```python
from build123d import *

# Parameters (mm, degrees)
SKETCH_1_R          = 2
SKETCH_1_R_2        = 11
SKETCH_1_R_3        = 13
EXTRUDE_1_DEPTH     = 5
SKETCH_1_4_R        = 13
SKETCH_1_4_R_2      = 11
CUT_EXTRUDE_1_DEPTH = 2


with BuildPart() as part:
    # Sketch 1 → Extrude 1 (new body)
    # profile 1 of 2: a face of its own
    with BuildSketch(Plane(origin=(0, 0, 0), x_dir=(1, 0, 0), z_dir=(0, 1, 0))):
        with BuildLine():
            ThreePointArc((-15, 22), (-14.414213562, 23.414213562), (-13, 24))
            Line((-13, 24), (13, 24))
            ThreePointArc((13, 24), (14.414213562, 23.414213562), (15, 22))
            Line((15, 22), (15, -22))
            ThreePointArc((15, -22), (14.414213562, -23.414213562), (13, -24))
            Line((13, -24), (-13, -24))
            ThreePointArc((-13, -24), (-14.414213562, -23.414213562), (-15, -22))
            Line((-15, -22), (-15, 0))
            Line((-15, 0), (-15, 22))
        make_face()
        with Locations(Location((0, -20, 0), (0, 0, 270))):
            Circle(SKETCH_1_R, mode=Mode.SUBTRACT)
        with Locations(Location((0, 20, 0), (0, 0, 270))):
            Circle(SKETCH_1_R, mode=Mode.SUBTRACT)
        with Locations(Location((0, 0, 0), (0, 0, 270))):
            Circle(SKETCH_1_R_2, mode=Mode.SUBTRACT)
    # profile 2 of 2: a face of its own
    with BuildSketch(Plane(origin=(0, 0, 0), x_dir=(1, 0, 0), z_dir=(0, 1, 0))):
        Circle(SKETCH_1_R_3)
        with Locations(Location((0, 0, 0), (0, 0, 270))):
            Circle(SKETCH_1_R_2, mode=Mode.SUBTRACT)
    extrude(amount=EXTRUDE_1_DEPTH)

    # Sketch 1_4 → Cut-Extrude 1 (cut)
    with BuildSketch(Plane(origin=(0, 0, 0), x_dir=(1, 0, 0), z_dir=(0, 1, 0))):
        with Locations(Location((0, 0, 0), (0, 0, 270))):
            Circle(SKETCH_1_4_R)
        with Locations(Location((0, 0, 0), (0, 0, 270))):
            Circle(SKETCH_1_4_R_2, mode=Mode.SUBTRACT)
    extrude(amount=CUT_EXTRUDE_1_DEPTH, mode=Mode.SUBTRACT)


solid = part.part
```
CAD build for the part. Positions are in the model's coordinates, mm. A direction names the side the tool comes from. Give positions to 0.01 mm unless a question says otherwise; leave off trailing zeros. Write each loop counter-clockwise with the first axis right and the second up, starting at its lowest first coordinate (ties: lowest second). Pieces come first, ordered by that corner, then holes. Notation, with made-up numbers: (2, 80.5) -> (33, 80.5) arc R14 ccw to (33, 95.5) -> close; hole circle Ø2 at (23.5, 25). An arc over 180 degrees is marked (long way). Write each question's results on one line, items separated by ' | '.
1. Cut at B-B, the plane x = 0. Write the cut outline in (y, z).
Geometry check:
outline: (0, -24) -> (5, -24) -> (5, -22) -> (0, -22) -> close; (0, -18) -> (5, -18) -> (5, -11) -> (2, -11) -> (2, -13) -> (0, -13) -> close; (0, 13) -> (2, 13) -> (2, 11) -> (5, 11) -> (5, 18) -> (0, 18) -> close; (0, 22) -> (5, 22) -> (5, 24) -> (0, 24) -> close
2. Cut at C-C, the plane y = 0.95. Write the cut outline in (x, z).
Geometry check:
outline: (-15, -22) arc R2 ccw to (-13, -24) -> (13, -24) arc R2 ccw to (15, -22) -> (15, 22) arc R2 ccw to (13, 24) -> (-13, 24) arc R2 ccw to (-15, 22) -> close; hole circle Ø26 at (0, 0); hole circle Ø4 at (0, -20); hole circle Ø4 at (0, 20)
3. Which spindle directions (+Z, -Z, +X, -X, +Y, -Y) get a long thin tool onto all of the face, cutting with end or side? Do faces 5 (the flat face through (3, 2, -11)), 6 (the flat face through (-15, 2, 0)). Say none if no direction does.
Geometry check:
face 5: -Y | face 6: +Z, -Z, -X, +Y, -Y
4. Wall check: probe 1 along Z at (x, y) = (-0.5, 4.5); probe 2 along X at (y, z) = (2, 20); probe 3 along X at (y, z) = (0.65, 0). Give the ranges that are in metal, low to high. Write a range as [from, to].
Geometry check:
probe 1: [-24, -21.94], [-18.06, -10.99], [10.99, 18.06], [21.94, 24] | probe 2: [-15, -2], [2, 15] | probe 3: [-15, -13], [13, 15]
5. Cut at A-A, the plane z = -20. Write the cut outline in (x, y).
Geometry check:
outline: (-15, 0) -> (-2, 0) -> (-2, 5) -> (-15, 5) -> close; (2, 0) -> (15, 0) -> (15, 5) -> (2, 5) -> close
6. Drop a flat-ended pin along its axis: P1, Ø1.5, axis at x = 11, z = 3.5, coming from the -Y side. Give the stop position or say it passes through.
Geometry check:
P1: y = 2
7. Cut at D-D, the plane z = 0. Write the cut outline in (x, y).
Geometry check:
outline: (-15, 0) -> (-13, 0) -> (-13, 2) -> (-11, 2) -> (-11, 5) -> (-15, 5) -> close; (11, 2) -> (13, 2) -> (13, 0) -> (15, 0) -> (15, 5) -> (11, 5) -> close
8. Two-plate mould, pull along Z, no slides. Class faces 1 (the cylindrical face through (-1.2, 2.5, 18.4)), 2 (the flat face through (0, 2, 24)), 3 (the cylindrical face through (-14.43, 2.46, -23.4)), 4 (the cylindrical face through (-10.74, 3.48, -2.38)): pulls with the +Z half, pulls with the -Z half, needs draft (parallel to the pull), parting line crosses it, or undercut.
Geometry check:
face 1: undercut | face 2: pulls with the +Z half | face 3: pulls with the -Z half | face 4: undercut
